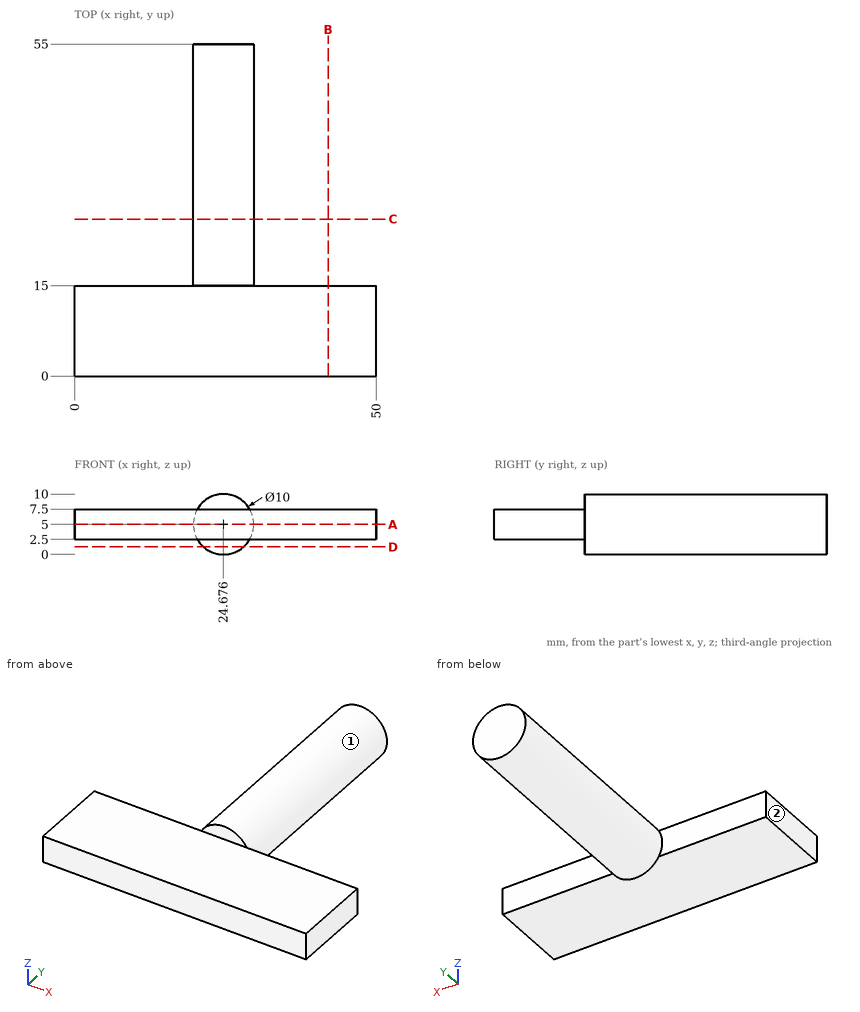
Input: dimensioned drawing with shaded views. Units: mm. Origin: part minimum x, y, z. A direction names the side the tool comes from. Give positions to 0.01 mm unless a question says otherwise; leave off trailing zeros. Loops run counter-clockwise (first coordinate to the right, second up) from the corner with the lowest first, then second, coordinate; pieces in that order, holes last. Notation, with made-up numbers: (57, -3) -> (103, -3) arc R17 cw to (103, 17) -> close; hole circle Ø5 at (13, 0). An arc over 180 degrees is marked (long way). Return JSON: item names as keys, results as strings.
Item 1: Access query for the marked faces 1 and 2. Directions: +Z, -Z, +X, -X, +Y, -Y. A direction counts if a zero-diameter tool reaches every point of the face in a straight line with its end or side. Return the directions, or none.
Filled in:
{"face 1": "+Y", "face 2": "+Z, -Z, -X, +Y, -Y"}
Item 2: Section A-A, the plane z = 5. Output: boundary loops of the cut face in (x, y), plus the area to 3 significant figures.
Filled in:
{"outline": "(0, 0) -> (50, 0) -> (50, 15) -> (29.68, 15) -> (29.68, 55) -> (19.68, 55) -> (19.68, 15) -> (0, 15) -> close", "area": "1,150 mm^2"}
Item 3: Section D-D, the plane z = 1.25. Output: boundary loops of the cut face in (x, y), plus the area to 3 significant figures.
Filled in:
{"outline": "(21.37, 15) -> (27.98, 15) -> (27.98, 55) -> (21.37, 55) -> close", "area": "265 mm^2"}
Item 4: Section B-B, the plane x = 42. Output: boundary loops of the cut face in (y, z).
Filled in:
{"outline": "(0, 2.5) -> (15, 2.5) -> (15, 7.5) -> (0, 7.5) -> close"}
Item 5: Section C-C, the plane y = 26. Output: boundary loops of the cut face in (x, z).
Filled in:
{"outline": "circle Ø10 at (24.68, 5)"}
Item 6: Line query: line 1 (Y direction, x = 36.5, z = 4.5); line 2 (Z direction, x = 12, y = 7); line 3 (X direction, y = 26.5, z = 4.75). Output: solid intervals per line, ascending.
Filled in:
{"line 1": "0 to 15", "line 2": "2.5 to 7.5", "line 3": "19.68 to 29.67"}
Item 7: Pin query (flat end, axial travel): P1, Ø1.3, axis at x = 23.5, z = 1, coming from the -Y side; P2, Ø1.5, axis at x = 38, z = 6.5, coming from the -Y side; P3, Ø4, axis at x = 40.5, z = 6, coming from the +Y side; P4, Ø4.5, axis at x = 20, y = 10, coming from the +Z side. Return the tip coordinate at first contact, or that it passes through.
Filled in:
{"P1": "y = 15", "P2": "y = 0", "P3": "y = 15", "P4": "z = 7.5"}
